Autodesk Inventor part; units mm, degrees
ref_plane "YZ Plane" through (0, 0, 0) normal (1, 0, 0) x (0, 1, 0)
ref_plane "XZ Plane" through (0, 0, 0) normal (0, 1, 0) x (-1, 0, 0)
ref_plane "XY Plane" through (0, 0, 0) normal (0, 0, 1) x (1, 0, 0)
sketch "Sketch1" plane through (0, 0, 0) normal (0, 0, 1) x (1, 0, 0)
  circle A0 centre (0, 0) radius 70
  line L0 (0, 0) -> (32.5, 0)
  circle A1 centre (32.5, 0) radius 3
  line L1 (0, 0) -> (0, 32.5)
  circle A2 centre (0, 32.5) radius 3
  circle A3 centre (-32.5, 0) radius 3
  circle A4 centre (0, -32.5) radius 3
  circle A5 centre (0, 0) radius 27
  dimension "d0" = 140
  dimension "d1" = 32.5
  dimension "d2" = 6
  dimension "d3" = 32.5
  dimension "d4" = 6
  dimension "d5" = 54
extrude "Extrusion1" add sketch "Sketch1" along normal blind 3.5
properties part number "Sprocket"
For this review, take the finished solid that the model builds, in its own axes (mm). Coordinates: 2 decimals unless noted, no trailing zeros. Order: outer loops, then holes, each group sorted by start corner. A loop starts at its lowest first (then second) coordinate and runs counter-clockwise, first axis right, second up. Notation, with made-up numbers: (12, 60.5) -> (49, 60.5) arc R19 cw to (49, 89.5) -> close; hole circle Ø11 at (-19.75, -37). An arc over 180 degrees is marked (long way). Answer as CSV lines item,"result".
Q1. We need section A-A (y = 0). State the section outline as (x, z) points, plus the area to 3 significant figures.
Model answer:
outline,"(-70, 0) -> (-35.5, 0) -> (-35.5, 3.5) -> (-70, 3.5) -> close; (-29.5, 0) -> (-27, 0) -> (-27, 3.5) -> (-29.5, 3.5) -> close; (27, 0) -> (29.5, 0) -> (29.5, 3.5) -> (27, 3.5) -> close; (35.5, 0) -> (70, 0) -> (70, 3.5) -> (35.5, 3.5) -> close"
area,"259 mm2"
Q2. Draft analysis for pull direction X (two halves, no side actions). For faces 1 (the face through (-55.55, 42.594, 1.726)), 2 (the face through (-2.21, -34.53, 1.73)), 3 (the face through (30, -15, 0)), state which applies: released by +X, released by -X, zero draft, split by the parting line, or undercut.
Model answer:
face 1,"split by the parting line"
face 2,"undercut"
face 3,"zero draft"
Q3. Wall thickness on line 1 along Y through (x, z) = (0, 0.85); line 2 along X through (y, z) = (-8, 0.2); line 3 along X through (y, z) = (17.5, 1.9): over which ranges is each line inside the solid? List them lowest first. Write a range as [from, to].
Model answer:
line 1,"y = [-70, -35.5], [-29.5, -27], [27, 29.5], [35.5, 70]"
line 2,"x = [-69.54, -25.79], [25.79, 69.54]"
line 3,"x = [-67.78, -20.56], [20.56, 67.78]"
Q4. We need section D-D (x = -32.5). State the section outline as (y, z) points.
Model answer:
outline,"(-62, 0) -> (-3, 0) -> (-3, 3.5) -> (-62, 3.5) -> close; (3, 0) -> (62, 0) -> (62, 3.5) -> (3, 3.5) -> close"
Q5. We need section C-C (z = 2.2). State the section outline as (x, y) points, plus the area to 3 significant figures.
Model answer:
outline,"circle Ø140 at (0, 0); hole circle Ø6 at (-32.5, 0); hole circle Ø54 at (0, 0); hole circle Ø6 at (0, -32.5); hole circle Ø6 at (0, 32.5); hole circle Ø6 at (32.5, 0)"
area,"13,000 mm2"
Q6. Clearance check with flat-ended pins moving along their axes: pin 1 Ø1 at (x, z) = (-9.5, 1.5) entering from +Y; pin 2 Ø1.5 at (x, z) = (28.5, 1.5) entering from -Y; pin 3 Ø2 at (y, z) = (-19, 2.5) entering from -X. State where each tip first meets the part, or that it passes through.
Model answer:
pin 1,"stops at y = 69.42"
pin 2,"stops at y = -64.26"
pin 3,"stops at x = -67.65"
